```python
from build123d import *

# Parameters (mm, degrees)
SKETCH1_W           = 22
SKETCH1_H           = 6
BOSS_EXTRUDE1_DEPTH = 1
BOSS_EXTRUDE2_DEPTH = 1
FILLET1_R           = 1


with BuildPart() as part:
    # Sketch1 → Boss-Extrude1 (new body)
    with BuildSketch(Plane(origin=(0, 0, 0), x_dir=(1, 0, 0), z_dir=(0, 1, 0))):
        Rectangle(SKETCH1_W, SKETCH1_H)
    extrude(amount=BOSS_EXTRUDE1_DEPTH)

    # Sketch2 → Boss-Extrude2 (add)
    with BuildSketch(Plane.XZ):
        with BuildLine():
            Line((11, 5), (-11, 5))
            ThreePointArc((-11, 5), (-12.414213562, 4.414213562), (-13, 3))
            Line((-13, 3), (-13, -3))
            ThreePointArc((-13, -3), (-12.414213562, -4.414213562), (-11, -5))
            Line((-11, -5), (11, -5))
            ThreePointArc((11, -5), (12.414213562, -4.414213562), (13, -3))
            Line((13, -3), (13, 3))
            ThreePointArc((13, 3), (12.414213562, 4.414213562), (11, 5))
        make_face()
    extrude(amount=BOSS_EXTRUDE2_DEPTH)

    # Fillet1
    fillet1_edges = [part.edges().sort_by_distance(p)[0] for p in [
        (11, 0.5, 3),
        (11, 0.5, -3),
        (-11, 0.5, -3),
        (-11, 0.5, 3),
    ]]
    fillet(fillet1_edges, radius=FILLET1_R)


solid = part.part
```
Build history of the part. All positions in model axes, mm. A direction names the side the tool comes from. Give positions to 0.01 mm unless a question says otherwise; leave off trailing zeros. Loops run counter-clockwise (first coordinate to the right, second up) from the corner with the lowest first, then second, coordinate; pieces in that order, holes last. Notation, with made-up numbers: (17.25, -6.75) - (68.25, -6.75) arc R21 ccw to (68.25, 31.25) - close; hole circle Ø3 at (20, 55). An arc over 180 degrees is marked (long way). Use a Markdown table: item, result.
(1) Wall check: line 1 along X through (y, z) = (0.45, -2); line 2 along Y through (x, z) = (2.75, 3.75); line 3 along Z through (x, y) = (-9.5, 0.4). Give the ranges that are in metal, low to high.
Taken from the geometry:
| item | result |
|---|---|
| line 1 | -11 to 11 |
| line 2 | -1 to 0 |
| line 3 | -3 to 3 |
(2) Drop a flat-ended pin along its axis: pin 1 Ø1 at (y, z) = (1, -2.5) entering from -X. Give the stop position or say it passes through.
Taken from the geometry:
| item | result |
|---|---|
| pin 1 | x = -11 |
(3) Band-saw the part on D-D (z = 3.25). Give the cut face in (x, y), and give its area (3 significant figures).
Taken from the geometry:
| item | result |
|---|---|
| outline | (-12.98, -1) - (12.98, -1) - (12.98, 0) - (-12.98, 0) - close |
| area | 26.0 mm2 |
(4) Which spindle directions (+Z, -Z, +X, -X, +Y, -Y) get a long thin tool onto all of the face, cutting with end or side? Do faces 1 (the face through (10.715, 0.507, 2.699)), 2 (the face through (10.699, 0.507, -2.715)), 3 (the face through (-10.715, 0.507, -2.699)), 4 (the face through (-0.1, 0.5, -3)). Say none if no direction does.
Taken from the geometry:
| item | result |
|---|---|
| face 1 | +Z, +X, +Y |
| face 2 | -Z, +X, +Y |
| face 3 | -Z, -X, +Y |
| face 4 | -Z, +X, -X, +Y |
(5) Band-saw the part on C-C (z = -4.5). Give the cut face in (x, y), and give its area (3 significant figures).
Taken from the geometry:
| item | result |
|---|---|
| outline | (-12.32, -1) - (12.32, -1) - (12.32, 0) - (-12.32, 0) - close |
| area | 24.6 mm2 |
(6) Band-saw the part on B-B (y = 0.35). Give the cut face in (x, z), and give its area (3 significant figures).
Taken from the geometry:
| item | result |
|---|---|
| outline | (-11, -2) arc R1 ccw to (-10, -3) - (10, -3) arc R1 ccw to (11, -2) - (11, 2) arc R1 ccw to (10, 3) - (-10, 3) arc R1 ccw to (-11, 2) - close |
| area | 131 mm2 |
(7) Band-saw the part on A-A (x = -7.5). Give the cut face in (y, z).
Taken from the geometry:
| item | result |
|---|---|
| outline | (-1, -5) - (0, -5) - (0, -3) - (1, -3) - (1, 3) - (0, 3) - (0, 5) - (-1, 5) - close |
